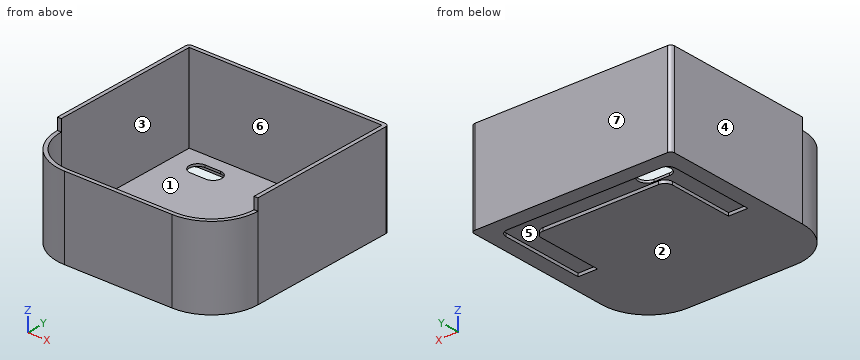
```python
from build123d import *

# Parameters (mm, degrees)
ESQUISSE2_W             = 260
ESQUISSE2_H             = 260
BOSS_EXTRU_1_DEPTH      = 120
CONG_1_R                = 60
CONG_2_R                = 5
ENL_V_MAT_EXTRU_1_DEPTH = 113
ESQUISSE4_W             = 260
ESQUISSE4_H             = 60
ENL_V_MAT_EXTRU_2_DEPTH = 15
ENL_V_MAT_EXTRU_3_DEPTH = 4
ENL_V_MAT_EXTRU_4_DEPTH = 10


with BuildPart() as part:
    # Esquisse2 → Boss.-Extru.1 (new body)
    with BuildSketch(Plane.XY):
        with Locations((130, 130)):
            Rectangle(ESQUISSE2_W, ESQUISSE2_H)
    extrude(amount=BOSS_EXTRU_1_DEPTH)

    # Congé1
    cong_1_edges = [part.edges().sort_by_distance(p)[0] for p in [
        (260, 0, 60),
        (0, 0, 60),
    ]]
    fillet(cong_1_edges, radius=CONG_1_R)

    # Congé2
    cong_2_edges = [part.edges().sort_by_distance(p)[0] for p in [
        (0, 260, 60),
        (260, 260, 60),
    ]]
    fillet(cong_2_edges, radius=CONG_2_R)

    # Esquisse3 → Enlèv. mat.-Extru.1 (cut)
    with BuildSketch(Plane.XY.offset(120)):
        with BuildLine():
            Line((5, 255), (255, 255))
            Line((255, 255), (255, 60))
            ThreePointArc((255, 60), (238.890872965, 21.109127035), (200, 5))
            Line((200, 5), (60, 5))
            ThreePointArc((60, 5), (21.109127035, 21.109127035), (5, 60))
            Line((5, 60), (5, 255))
        make_face()
    extrude(amount=-ENL_V_MAT_EXTRU_1_DEPTH, mode=Mode.SUBTRACT)

    # Esquisse4 → Enlèv. mat.-Extru.2 (cut)
    with BuildSketch(Plane.XY.offset(120)):
        with Locations((130, 30)):
            Rectangle(ESQUISSE4_W, ESQUISSE4_H)
    extrude(amount=-ENL_V_MAT_EXTRU_2_DEPTH, mode=Mode.SUBTRACT)

    # Esquisse5 → Enlèv. mat.-Extru.3 (cut)
    with BuildSketch(Plane(origin=(0, 0, 0), x_dir=(-1, 0, 0), z_dir=(0, 0, -1))):
        with BuildLine():
            Line((-240, 120), (-240, 230))
            ThreePointArc((-240, 230), (-237.071067812, 237.071067812), (-230, 240))
            Line((-230, 240), (-30, 240))
            ThreePointArc((-30, 240), (-22.928932188, 237.071067812), (-20, 230))
            Line((-20, 230), (-20, 120))
            Line((-20, 120), (-45, 120))
            Line((-45, 120), (-45, 205))
            ThreePointArc((-45, 205), (-47.928932188, 212.071067812), (-55, 215))
            Line((-55, 215), (-205, 215))
            ThreePointArc((-205, 215), (-212.071067812, 212.071067812), (-215, 205))
            Line((-215, 205), (-215, 120))
            Line((-215, 120), (-240, 120))
        make_face()
    extrude(amount=-ENL_V_MAT_EXTRU_3_DEPTH, mode=Mode.SUBTRACT)

    # Esquisse6 → Enlèv. mat.-Extru.4 (cut)
    with BuildSketch(Plane(origin=(0, 0, 4), x_dir=(-1, 0, 0), z_dir=(0, 0, -1))):
        with BuildLine():
            Line((-39.5, 238.5), (-59.5, 238.5))
            ThreePointArc((-59.5, 238.5), (-70.5, 227.5), (-59.5, 216.5))
            Line((-59.5, 216.5), (-39.5, 216.5))
            ThreePointArc((-39.5, 216.5), (-28.5, 227.5), (-39.5, 238.5))
        make_face()
    extrude(amount=-ENL_V_MAT_EXTRU_4_DEPTH, mode=Mode.SUBTRACT)


solid = part.part
```
Design review of the part built by this model. Coordinates are the model's own, in mm. Face numbers are marked on the shaded views. A direction names the side the tool comes from. Coordinates: 2 decimals unless noted, no trailing zeros. Loops run counter-clockwise (first coordinate to the right, second up) from the corner with the lowest first, then second, coordinate; pieces in that order, holes last. Notation, with made-up numbers: M -31,44 L 8,44 A24 ccw 8,78 Z; hole C 0.25,83.5 d4. An arc over 180 degrees is marked long. One line per question, with ' | ' between items.
(1) We need section B-B (x = 109). Give the boundary of the cut face in (y, z).
Filled in:
outline: M 0,0 L 215,0 L 215,4 L 240,4 L 240,0 L 260,0 L 260,120 L 255,120 L 255,7 L 5,7 L 5,105 L 0,105 Z
(2) We need section D-D (y = 179.5). Give the boundary of the cut face in (x, z), and give its area (3 significant figures).
Filled in:
outline: M 0,0 L 20,0 L 20,4 L 45,4 L 45,0 L 215,0 L 215,4 L 240,4 L 240,0 L 260,0 L 260,120 L 255,120 L 255,7 L 5,7 L 5,120 L 0,120 Z | area: 2,750 mm^2
(3) We need section A-A (y = 116.5). Give the boundary of the cut face in (x, z), and give its area (3 significant figures).
Filled in:
outline: M 0,0 L 260,0 L 260,120 L 255,120 L 255,7 L 5,7 L 5,120 L 0,120 Z | area: 2,950 mm^2
(4) For pin 1 Ø5.5 at (x, z) = (256.5, 114.5) entering from -Y; pin 2 Ø3 at (x, y) = (232, 142) entering from -Z; pin 3 Ø18 at (x, y) = (146, 19) entering from +Z, all flat-tipped, find the tip position at first contact; note any pin that passes through.
Filled in:
pin 1: stops at y = 60 | pin 2: stops at z = 4 | pin 3: stops at z = 7
(5) We need section C-C (z = 78.5). Give the boundary of the cut face in (x, y).
Filled in:
outline: M 0,60 A60 ccw 60,0 L 200,0 A60 ccw 260,60 L 260,255 A5 ccw 255,260 L 5,260 A5 ccw 0,255 Z; hole M 5,60 A55 ccw 60,5 L 200,5 A55 ccw 255,60 L 255,255 L 5,255 Z
(6) Wall thickness on probe 1 along Y at (x, z) = (186.5, 66.5); probe 2 along Z at (x, y) = (162, 71.5): over which ranges is each line inside the solid? List them lowest first.
Filled in:
probe 1: y = 0 to 5, 255 to 260 | probe 2: z = 0 to 7
(7) Machinability: for the marked faces 5, 6 and 7, which of the approach directions +Z, -Z, +X, -X, +Y, -Y give a long, thin tool a straight path to every point of the face, cutting with its end or side? Answer none if there is none.
Filled in:
face 5: -Z | face 6: +Z | face 7: +Z, -Z, +X, -X, +Y
(8) Draft analysis for pull direction X (two halves, no side actions). For the marked faces 1, 2, 3 and 4, state which applies: released by +X, released by -X, zero draft, split by the parting line, or undercut.
Filled in:
face 1: undercut | face 2: zero draft | face 3: undercut | face 4: released by -X
